The figure shows three views and two pictorial views of one solid part (mm, origin at its lowest corner). Answer the questions. A direction names the side the tool comes from. Round coordinates to 2 decimals unless told otherwise and drop trailing zeros. Write each loop counter-clockwise with the first axis right and the second up, starting at its lowest first coordinate (ties: lowest second). Pieces come first, ordered by that corner, then holes. Notation, with made-up numbers: M 74.5,39.5 L 117.5,39.5 A23 ccw 117.5,78.5 Z; hole C -9,17 d10. An arc over 180 degrees is marked long. One line per item, written item: value. Start each with the question number.
Q1. Consider probe 1 along Y at (x, z) = (55, 103.5); probe 2 along X at (y, z) = (4.5, 30); probe 3 along Z at (x, y) = (4, 12.5). Determine where each line is inside the solid, lowest interval first.
Q2. Find section C-C (y = 16.5). Write down the section's boundary in (x, z), and give its area (3 significant figures).
Q3. Find section D-D (x = 20). Write down the section's boundary in (y, z).
Q4. Find section B-B (z = 40.5). Write down the section's boundary in (x, y), and give its area (3 significant figures).
Q5. A tool of negligible diameter and unlimited length cuts with its end or side. For the marked faces 1 and 2, from which of +Z, -Z, +X, -X, +Y, -Y can it reach the whole face along a straight path? Write none if from no direction.
Q6. Given pin 1 Ø3 at (y, z) = (14.5, 105) entering from +X; pin 2 Ø10 at (x, y) = (34.5, 8.5) entering from -Z; pin 3 Ø5 at (x, y) = (13.5, 15.5) entering from -Z, each flat-ended and moving along its own axis, determine where each tip first touches the part or whether it passes through.
Q7. Find section A-A (x = 7). Write down the section's boundary in (y, z).
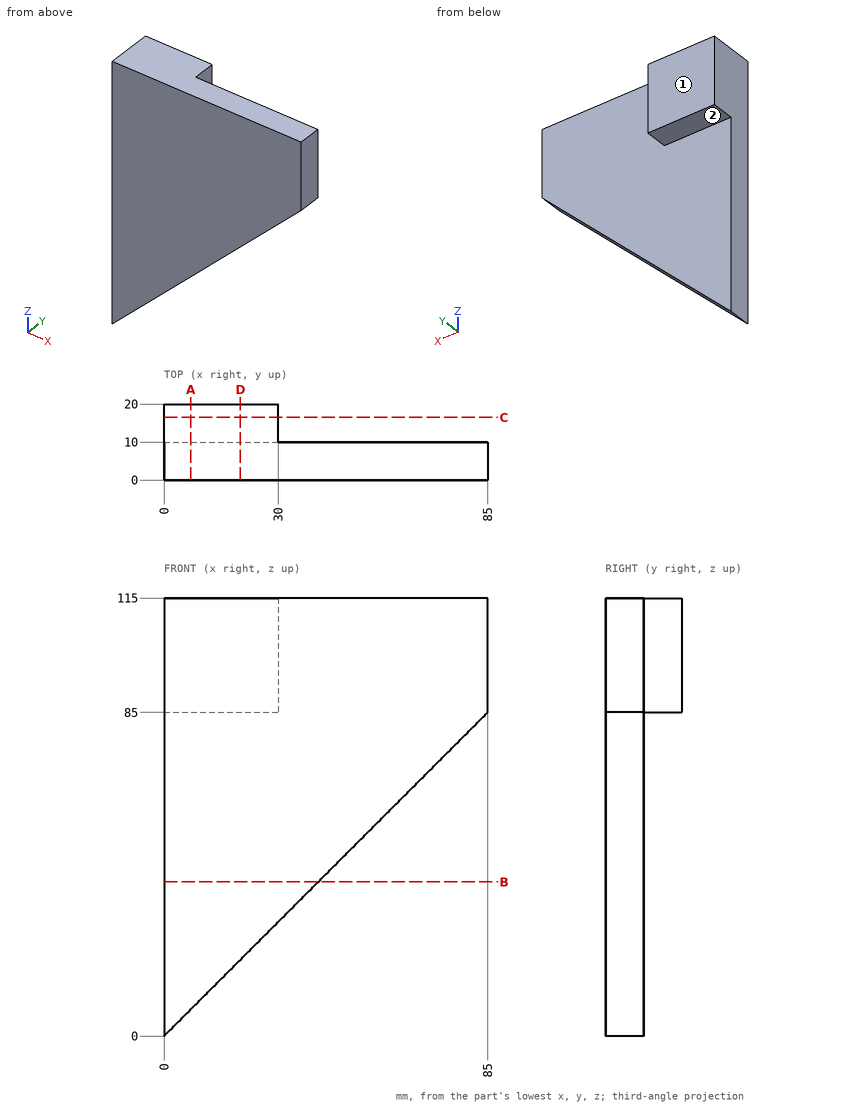
The answers:
1. probe 1: 0 to 10
1. probe 2: 0 to 30
1. probe 3: 85 to 115
2. outline: M 0,85 L 30,85 L 30,115 L 0,115 Z
2. area: 900 mm2
3. outline: M 0,20 L 10,20 L 10,85 L 20,85 L 20,115 L 0,115 Z
4. outline: M 0,0 L 40.5,0 L 40.5,10 L 0,10 Z
4. area: 405 mm2
5. face 1: +Z, -Z, +X, -X, +Y
5. face 2: -Z, +X, -X, +Y
6. pin 1: x = 30
6. pin 2: z = 29.5
6. pin 3: z = 85
7. outline: M 0,7 L 10,7 L 10,85 L 20,85 L 20,115 L 0,115 Z
